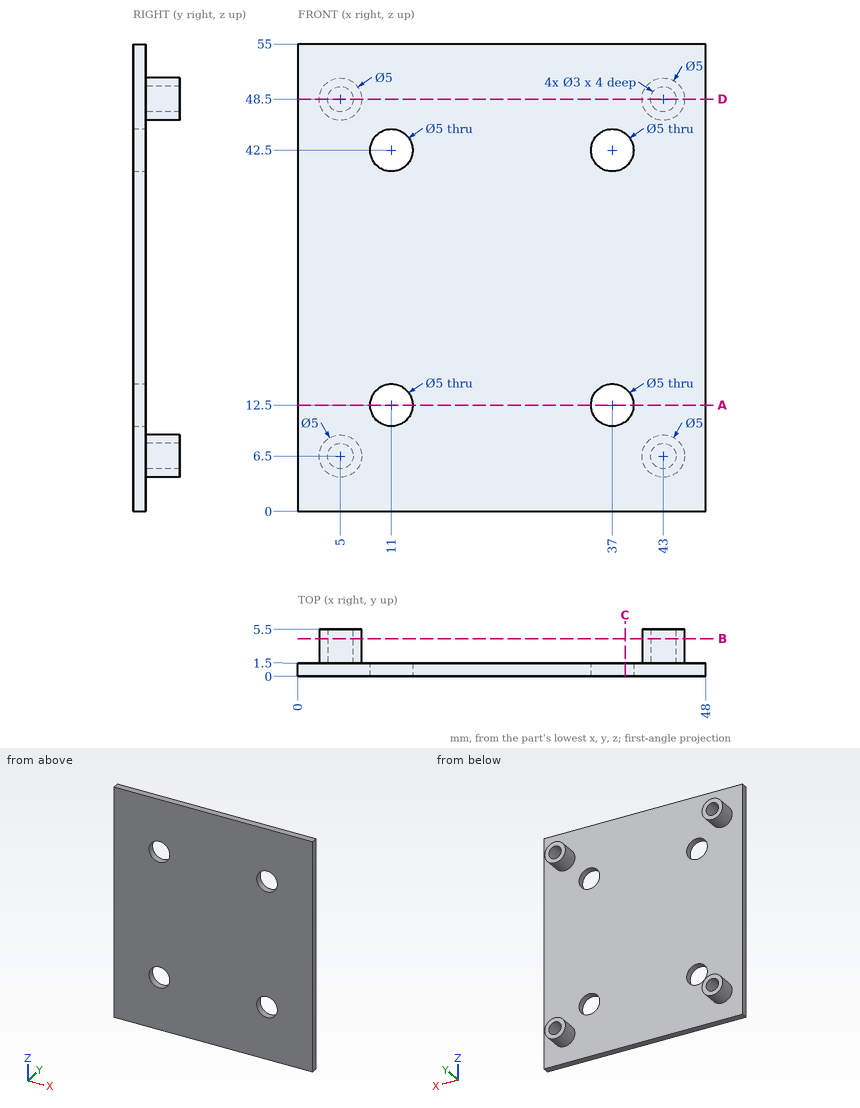
Part print with two shaded views. Sizes in mm from the minimum x, y, z corner. Coordinates: 2 decimals unless noted, no trailing zeros. Order: outer loops, then holes, each group sorted by start corner. A loop starts at its lowest first (then second) coordinate and runs counter-clockwise, first axis right, second up. Notation, with made-up numbers: M 23,-33 L 31,-33 A15 ccw 31,-4 Z; hole C 76,41 d3. An arc over 180 degrees is marked long. One line per question, with ' | ' between items. Start each with the question number.
1. Cut at A-A (z = 12.5). Write the cut outline in (x, y), plus the area to 3 significant figures.
2. Cut at B-B (y = 4.4). Write the cut outline in (x, z), plus the area to 3 significant figures.
3. Flat gauge pins, fed straight in: P1, Ø4, axis at x = 25.5, z = 48, coming from the +Y side; P2, Ø1.5, axis at x = 39.5, y = 3.5, coming from the +Z side. Where does each tip first touch, or does it go through?
4. Cut at D-D (z = 48.5). Write the cut outline in (x, y).
5. Cut at C-C (x = 38.5). Write the cut outline in (y, z), plus the area to 3 significant figures.
6. Wall check: line 1 along X through (y, z) = (0.75, 12.5); line 2 along X through (y, z) = (2.95, 48.5); line 3 along Z through (x, y) = (11, 1.2). Give the ranges that are in metal, low to high. Write a range as [from, to].
The answers:
1) outline: M 0,0 L 8.5,0 L 8.5,1.5 L 0,1.5 Z; M 13.5,0 L 34.5,0 L 34.5,1.5 L 13.5,1.5 Z; M 39.5,0 L 48,0 L 48,1.5 L 39.5,1.5 Z | area: 57.0 mm2
2) outline: C 5,6.5 d5; C 5,48.5 d5; C 43,6.5 d5; C 43,48.5 d5; hole C 5,6.5 d3; hole C 5,48.5 d3; hole C 43,6.5 d3; hole C 43,48.5 d3 | area: 50.3 mm2
3) P1: stops at y = 1.5 | P2: passes through
4) outline: M 0,0 L 48,0 L 48,1.5 L 45.5,1.5 L 45.5,5.5 L 44.5,5.5 L 44.5,1.5 L 41.5,1.5 L 41.5,5.5 L 40.5,5.5 L 40.5,1.5 L 7.5,1.5 L 7.5,5.5 L 6.5,5.5 L 6.5,1.5 L 3.5,1.5 L 3.5,5.5 L 2.5,5.5 L 2.5,1.5 L 0,1.5 Z
5) outline: M 0,0 L 1.5,0 L 1.5,10.5 L 0,10.5 Z; M 0,14.5 L 1.5,14.5 L 1.5,40.5 L 0,40.5 Z; M 0,44.5 L 1.5,44.5 L 1.5,55 L 0,55 Z | area: 70.5 mm2
6) line 1: x = [0, 8.5], [13.5, 34.5], [39.5, 48] | line 2: x = [2.5, 3.5], [6.5, 7.5], [40.5, 41.5], [44.5, 45.5] | line 3: z = [0, 10], [15, 40], [45, 55]
